Can you work these out from the model? Positions are in its coordinate system, mm. Face numbers are marked on the shaded views. A direction names the side the tool comes from. Round coordinates to 2 decimals unless told otherwise and drop trailing zeros. Order: outer loops, then holes, each group sorted by start corner. A loop starts at its lowest first (then second) coordinate and runs counter-clockwise, first axis right, second up. Notation, with made-up numbers: (7.25, -29.75) -> (16.25, -29.75) arc R31 cw to (16.25, -3.75) -> close; hole circle Ø5 at (20, 55.5). An arc over 180 degrees is marked (long way). Use a Markdown table: item, result. Add a question column.
Q1. If we section it at D-D on x = 10: List the corners of the cut face in (y, z) for me, plus the area to 3 significant figures.
Q2. I need wall thicknesses on line 1 along Y through (x, z) = (16, 5.25); line 2 along Y through (x, z) = (-22.5, 0.8); line 3 along X through (y, z) = (12.5, 6.5). Which ranges of each line are inside material? Lowest first, please. Write a range as [from, to].
Q3. We'd pull the mould along X, two halves only. Please class the marked faces 1, 2, 3 and 4: +X half, -X half, draft (parallel to the pull), parting line (faces both ways), or undercut.
Q4. For the marked faces 5, 6 and 7, which set-ups out of +Z, -Z, +X, -X, +Y, -Y let a thin tool reach every point of the face, with its end or its side?
Q5. I'm going to push flat-ended pins straight in: pin 1 Ø5 at (y, z) = (-2.5, 11.5) entering from +X; pin 2 Ø15.5 at (x, y) = (8, -4) entering from +Z; pin 3 Ø1.7 at (x, y) = (19.5, -3.5) entering from +Z; pin 4 Ø2.5 at (x, y) = (-22.5, 0) entering from +Z. Where does each tip first touch, or does it pass through?
Q6. If we section it at C-C on y = 13: List the corners of the cut face in (x, z) for me.
Q7. If we section it at B-B on z = 15.5: List the corners of the cut face in (x, y) for me, plus the area to 3 significant figures.
Q8. If we section it at A-A on y = 0: List the corners of the cut face in (x, z) for me.
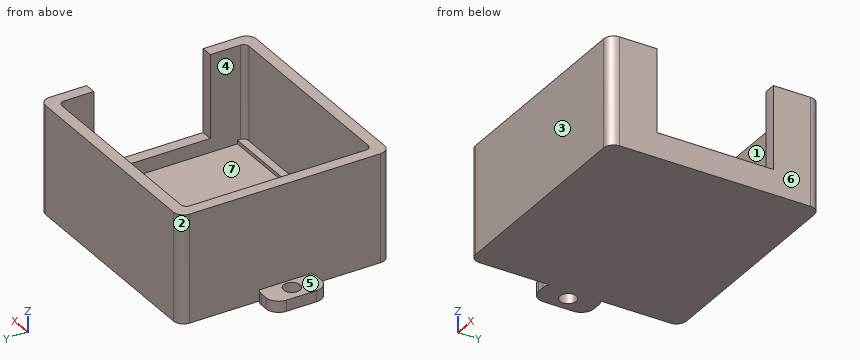
```python
from build123d import *

# Parameters (mm, degrees)
FACTORY_ABS_FLOOR_41X38_DEPTH       = 2
FACTORY_ABS_SIDEWALLS_START         = 2
FACTORY_ABS_SIDEWALLS_DEPTH         = 17.5
FACTORY_TERMINAL_OPENING_START      = 4.5
FACTORY_TERMINAL_OPENING_SKETCH_W   = 3.2
FACTORY_TERMINAL_OPENING_SKETCH_H   = 21
FACTORY_TERMINAL_OPENING_DEPTH      = 15
FACTORY_MOUNTING_EAR_DEPTH          = 2
FACTORY_EAR_REFERENCE_HOLE_SKETCH_R = 1.5
FACTORY_EAR_REFERENCE_HOLE_DEPTH    = 2
PCB_SUPPORT_LEDGES_START            = 2
PCB_SUPPORT_LEDGES_SKETCH_W         = 36.9
PCB_SUPPORT_LEDGES_SKETCH_H         = 1.4
PCB_SUPPORT_LEDGES_DEPTH            = 0.65


with BuildPart() as part:
    # Factory_ABS_floor_41x38_Sketch → Factory_ABS_floor_41x38 (new body)
    with BuildSketch(Plane.XY):
        with BuildLine():
            Line((-18.7, -19), (18.7, -19))
            ThreePointArc((18.7, -19), (19.972792206, -18.472792206), (20.5, -17.2))
            Line((20.5, -17.2), (20.5, 17.2))
            ThreePointArc((20.5, 17.2), (19.972792206, 18.472792206), (18.7, 19))
            Line((18.7, 19), (-18.7, 19))
            ThreePointArc((-18.7, 19), (-19.972792206, 18.472792206), (-20.5, 17.2))
            Line((-20.5, 17.2), (-20.5, -17.2))
            ThreePointArc((-20.5, -17.2), (-19.972792206, -18.472792206), (-18.7, -19))
        make_face()
    extrude(amount=FACTORY_ABS_FLOOR_41X38_DEPTH)

    # Factory_ABS_sidewalls_Sketch → Factory_ABS_sidewalls (add)
    with BuildSketch(Plane.XY.offset(FACTORY_ABS_SIDEWALLS_START)):
        with BuildLine():
            Line((-18.7, -19), (18.7, -19))
            ThreePointArc((18.7, -19), (19.972792206, -18.472792206), (20.5, -17.2))
            Line((20.5, -17.2), (20.5, 17.2))
            ThreePointArc((20.5, 17.2), (19.972792206, 18.472792206), (18.7, 19))
            Line((18.7, 19), (-18.7, 19))
            ThreePointArc((-18.7, 19), (-19.972792206, 18.472792206), (-20.5, 17.2))
            Line((-20.5, 17.2), (-20.5, -17.2))
            ThreePointArc((-20.5, -17.2), (-19.972792206, -18.472792206), (-18.7, -19))
        make_face()
        with BuildLine():
            Line((-17.4, -16.9), (17.4, -16.9))
            ThreePointArc((17.4, -16.9), (18.107106781, -16.607106781), (18.4, -15.9))
            Line((18.4, -15.9), (18.4, 15.9))
            ThreePointArc((18.4, 15.9), (18.107106781, 16.607106781), (17.4, 16.9))
            Line((17.4, 16.9), (-17.4, 16.9))
            ThreePointArc((-17.4, 16.9), (-18.107106781, 16.607106781), (-18.4, 15.9))
            Line((-18.4, 15.9), (-18.4, -15.9))
            ThreePointArc((-18.4, -15.9), (-18.107106781, -16.607106781), (-17.4, -16.9))
        make_face(mode=Mode.SUBTRACT)
    extrude(amount=FACTORY_ABS_SIDEWALLS_DEPTH)

    # Factory_terminal_opening_Sketch → Factory_terminal_opening (cut)
    with BuildSketch(Plane.XY.offset(FACTORY_TERMINAL_OPENING_START)):
        with Locations((19.8, 0)):
            Rectangle(FACTORY_TERMINAL_OPENING_SKETCH_W, FACTORY_TERMINAL_OPENING_SKETCH_H)
    extrude(amount=FACTORY_TERMINAL_OPENING_DEPTH, mode=Mode.SUBTRACT)

    # Factory_mounting_ear_Sketch → Factory_mounting_ear (add)
    with BuildSketch(Plane.XY):
        with BuildLine():
            Line((-23, -5), (-21.7, -5))
            ThreePointArc((-21.7, -5), (-20.073654403, -4.326345597), (-19.4, -2.7))
            Line((-19.4, -2.7), (-19.4, 2.7))
            ThreePointArc((-19.4, 2.7), (-20.073654403, 4.326345597), (-21.7, 5))
            Line((-21.7, 5), (-23, 5))
            ThreePointArc((-23, 5), (-24.626345597, 4.326345597), (-25.3, 2.7))
            Line((-25.3, 2.7), (-25.3, -2.7))
            ThreePointArc((-25.3, -2.7), (-24.626345597, -4.326345597), (-23, -5))
        make_face()
    extrude(amount=FACTORY_MOUNTING_EAR_DEPTH)

    # Factory_ear_reference_hole_Sketch → Factory_ear_reference_hole (cut)
    with BuildSketch(Plane.XY):
        with Locations((-22.5, 0)):
            Circle(FACTORY_EAR_REFERENCE_HOLE_SKETCH_R)
    extrude(amount=FACTORY_EAR_REFERENCE_HOLE_DEPTH, mode=Mode.SUBTRACT)

    # PCB_support_ledges_Sketch → PCB_support_ledges (add)
    with BuildSketch(Plane.XY.offset(PCB_SUPPORT_LEDGES_START)):
        with Locations((0, -16.1)):
            Rectangle(PCB_SUPPORT_LEDGES_SKETCH_W, PCB_SUPPORT_LEDGES_SKETCH_H)
        with Locations((0, 16.1)):
            Rectangle(PCB_SUPPORT_LEDGES_SKETCH_W, PCB_SUPPORT_LEDGES_SKETCH_H)
    extrude(amount=PCB_SUPPORT_LEDGES_DEPTH)


solid = part.part
```
Answer below:
| question | item | result |
|---|---|---|
| 1 | outline | (-19, 0) -> (19, 0) -> (19, 19.5) -> (16.9, 19.5) -> (16.9, 2) -> (16.8, 2) -> (16.8, 2.65) -> (15.4, 2.65) -> (15.4, 2) -> (-15.4, 2) -> (-15.4, 2.65) -> (-16.8, 2.65) -> (-16.8, 2) -> (-16.9, 2) -> (-16.9, 19.5) -> (-19, 19.5) -> close |
| 1 | area | 151 mm² |
| 2 | line 1 | [-19, -16.9], [16.9, 19] |
| 2 | line 2 | [-5, -1.5], [1.5, 5] |
| 2 | line 3 | [-20.5, -18.4], [18.4, 20.5] |
| 3 | face 1 | undercut |
| 3 | face 2 | -X half |
| 3 | face 3 | draft |
| 3 | face 4 | undercut |
| 4 | face 5 | +Z, -X, +Y, -Y |
| 4 | face 6 | +Z, -Z, +X, +Y, -Y |
| 4 | face 7 | +Z |
| 5 | pin 1 | x = -18.4 |
| 5 | pin 2 | z = 2 |
| 5 | pin 3 | z = 4.5 |
| 5 | pin 4 | through |
| 6 | outline | (-20.5, 0) -> (20.5, 0) -> (20.5, 19.5) -> (18.4, 19.5) -> (18.4, 2) -> (-18.4, 2) -> (-18.4, 19.5) -> (-20.5, 19.5) -> close |
| 7 | outline | (-20.5, -17.2) arc R1.8 ccw to (-18.7, -19) -> (18.7, -19) arc R1.8 ccw to (20.5, -17.2) -> (20.5, -10.5) -> (18.4, -10.5) -> (18.4, -15.9) arc R1 cw to (17.4, -16.9) -> (-17.4, -16.9) arc R1 cw to (-18.4, -15.9) -> (-18.4, 15.9) arc R1 cw to (-17.4, 16.9) -> (17.4, 16.9) arc R1 cw to (18.4, 15.9) -> (18.4, 10.5) -> (20.5, 10.5) -> (20.5, 17.2) arc R1.8 ccw to (18.7, 19) -> (-18.7, 19) arc R1.8 ccw to (-20.5, 17.2) -> close |
| 7 | area | 268 mm² |
| 8 | outline | (-25.3, 0) -> (-24, 0) -> (-24, 2) -> (-25.3, 2) -> close; (-21, 0) -> (20.5, 0) -> (20.5, 4.5) -> (18.4, 4.5) -> (18.4, 2) -> (-18.4, 2) -> (-18.4, 19.5) -> (-20.5, 19.5) -> (-20.5, 2) -> (-21, 2) -> close |
